Verification items for this drawing (mm, ordinates from the low corner). A direction names the side the tool comes from. Coordinates: 2 decimals unless noted, no trailing zeros. Order: outer loops, then holes, each group sorted by start corner. A loop starts at its lowest first (then second) coordinate and runs counter-clockwise, first axis right, second up. Notation, with made-up numbers: (-2, -13.75) -> (13, -13.75) arc R20 ccw to (13, 5.25) -> close; hole circle Ø4 at (19.25, -26). An arc over 180 degrees is marked (long way). Answer in a Markdown table with one row per item. Add a question column.
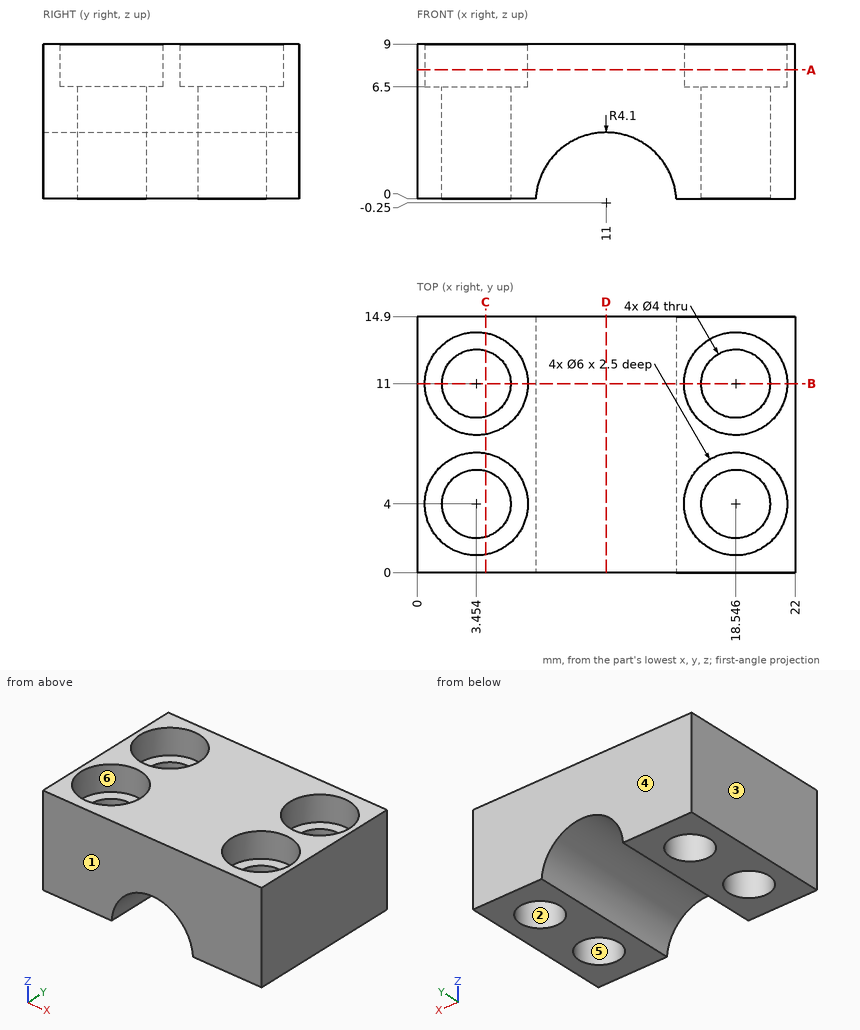
(1) Mould release check, pull along Y, two halves, no side actions. Record for the marked faces 1, 2, 3 and 4: +Y half, -Y half, draft (parallel to the pull), parting line (faces both ways), or undercut.
(2) Cross-section at B-B (y = 11). Enter the section's corners in (x, z).
(3) Cross-section at C-C (x = 4). Enter the section's corners in (y, z).
(4) Access from +Z, -Z, +X, -X, +Y, -Y to the whole of each face (thin tool, end or side, straight path). Record for the marked faces 5 and 6.
(5) Scan lines: line 1 along X through (y, z) = (3.25, 4); line 2 along Y through (x, z) = (18.25, 7) (1 decimal); line 3 along Z through (x, y) = (5, 6.5). Record each from-to range of solid material in increasing order.
(6) Go/stop test with flat-tipped pins: P1, Ø5, axis at x = 3.45, y = 11, coming from the +Z side; P2, Ø5, axis at x = 18.55, y = 4, coming from the -Z side; P3, Ø2.5, axis at x = 3.45, y = 4, coming from the +Z side. Record where each tip stops, or that it passes through.
(7) Cross-section at D-D (x = 11). Enter the section's corners in (y, z).
(8) Cross-section at A-A (z = 7.5). Enter the section's corners in (x, y), plus the area to 3 significant figures.
Checks:
| question | item | result |
|---|---|---|
| 1 | face 1 | -Y half |
| 1 | face 2 | undercut |
| 1 | face 3 | draft |
| 1 | face 4 | +Y half |
| 2 | outline | (0, 0) -> (1.45, 0) -> (1.45, 6.5) -> (0.45, 6.5) -> (0.45, 9) -> (0, 9) -> close; (5.45, 0) -> (6.91, 0) arc R4.1 cw to (15.09, 0) -> (16.55, 0) -> (16.55, 6.5) -> (15.55, 6.5) -> (15.55, 9) -> (6.45, 9) -> (6.45, 6.5) -> (5.45, 6.5) -> close; (20.55, 0) -> (22, 0) -> (22, 9) -> (21.55, 9) -> (21.55, 6.5) -> (20.55, 6.5) -> close |
| 3 | outline | (0, 0) -> (2.08, 0) -> (2.08, 6.5) -> (1.05, 6.5) -> (1.05, 9) -> (0, 9) -> close; (5.92, 0) -> (9.08, 0) -> (9.08, 6.5) -> (8.05, 6.5) -> (8.05, 9) -> (6.95, 9) -> (6.95, 6.5) -> (5.92, 6.5) -> close; (12.92, 0) -> (14.9, 0) -> (14.9, 9) -> (13.95, 9) -> (13.95, 6.5) -> (12.92, 6.5) -> close |
| 4 | face 5 | +Z, -Z |
| 4 | face 6 | +Z |
| 5 | line 1 | 0 to 1.6, 5.31 to 16.69, 20.4 to 22 |
| 5 | line 2 | 0 to 1, 7 to 8, 14 to 14.9 |
| 5 | line 3 | 0 to 6.5 |
| 6 | P1 | z = 6.5 |
| 6 | P2 | z = 0 |
| 6 | P3 | through |
| 7 | outline | (0, 3.85) -> (14.9, 3.85) -> (14.9, 9) -> (0, 9) -> close |
| 8 | outline | (0, 0) -> (22, 0) -> (22, 14.9) -> (0, 14.9) -> close; hole circle Ø6 at (3.45, 4); hole circle Ø6 at (3.45, 11); hole circle Ø6 at (18.55, 4); hole circle Ø6 at (18.55, 11) |
| 8 | area | 215 mm² |
